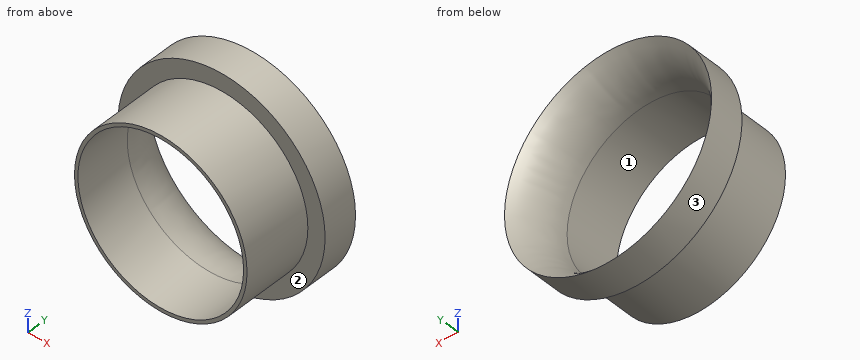
from build123d import *

# Parameters (mm, degrees)
F0_R     = 30
F1_DEPTH = 50
F2_R     = 30
F2_R_2   = 25
F3_DEPTH = 40
F4_R     = 24
F5_DEPTH = 60
F7_DEPTH = 20


# Not quite as in the source:
# - a fillet or chamfer that OpenCascade refuses, or shapes differently, is made with other operations: its cross-section is extruded or revolved along the edge and cut away or added


with BuildPart() as f1:
    # F0 (on Front) → F1 (new body)
    with BuildSketch(Plane.XZ):
        Circle(F0_R)
    extrude(amount=-F1_DEPTH)

    # F2 (on face) → F3 (cut)
    with BuildSketch(Plane.XZ):
        Circle(F2_R)
        Circle(F2_R_2, mode=Mode.SUBTRACT)
    extrude(amount=-F3_DEPTH, mode=Mode.SUBTRACT)

    # F4 (on face) → F5 (cut)
    with BuildSketch(Plane.XZ):
        Circle(F4_R)
    extrude(amount=-F5_DEPTH, mode=Mode.SUBTRACT)

    # F6: fillet of radius 18.8308657865 on 1 edges, made by hand

    # F6_s1 → F6_t2 (revolve, cut)
    with BuildSketch(Plane.XY):
        with BuildLine():
            ThreePointArc((30, 50), (25.5650351112, 43.7331811345), (24, 36.2170253777))
            Line((24, 36.2170253777), (23.6233826843, 36.2170253777))
            Line((23.6233826843, 36.2170253777), (23.6233826843, 50))
            Line((23.6233826843, 50), (24, 50.3766173157))
            ThreePointArc((24, 50.3766173157), (27, 50.3766173157), (29.7433826843, 50.2756594924))
            Line((29.7433826843, 50.2756594924), (30, 50))
        make_face()
    revolve(axis=Axis((0, 50, 0), (0, -1, 0)), mode=Mode.SUBTRACT)

    # F7 (cut): a face of the model
    f7_faces = [f1.faces().sort_by_distance(p)[0] for p in [
        (-24.2928932188, 0, 0),
    ]]
    extrude(f7_faces, amount=-F7_DEPTH, mode=Mode.SUBTRACT)


solid = f1.part
Geometry check sheet. Reference: the model listing, model coordinates, mm. Face numbers are marked on the shaded views. Round coordinates to 2 decimals unless told otherwise and drop trailing zeros. Loops run counter-clockwise (first coordinate to the right, second up) from the corner with the lowest first, then second, coordinate; pieces in that order, holes last.
Item 1: Cross-section at C-C on y = 34.25. Record the boundary of the cut face in (x, z).
Item 2: Cross-section at D-D on y = 38.25. Record the boundary of the cut face in (x, z).
Item 3: Mould release check, pull along Z, two halves, no side actions. Record for the marked faces 1, 2 and 3: pulls with the +Z half, pulls with the -Z half, needs draft (parallel to the pull), parting line crosses it, or undercut.
Item 4: Cross-section at A-A on z = 0. Record the boundary of the cut face in (x, y), then the cut area to 3 significant figures.
Item 5: Cross-section at B-B on x = 0. Record the boundary of the cut face in (y, z).
Item 6: Gauge pin test, flat ends, axial feed: pin 1 (6 mm diameter, centred on y = 42, z = -11.5, fed in from -X); pin 2 (2 mm diameter, centred on x = 4.5, y = 32.5, fed in from -Z); pin 3 (4 mm diameter, centred on x = -19.5, z = 9, fed in from -Y); pin 4 (5 mm diameter, centred on y = 46.5, z = 19, fed in from -X). Record the tip position at first contact, or that the pin passes through.
Item 7: Thickness scan on line 1 (Z direction, x = 0, y = 30.75); line 2 (Z direction, x = -12, y = 36.25); line 3 (X direction, y = 32.5, z = 15) (3 decimals). Record the ranges inside material, lowest first.
Answer sheet:
1. outline: circle Ø50 at (0, 0); hole circle Ø48 at (0, 0)
2. outline: circle Ø50 at (0, 0); hole circle Ø48.22 at (0, 0)
3. face 1: undercut
3. face 2: needs draft
3. face 3: parting line crosses it
4. outline: (-30, 40) - (-25, 40) - (-25, 20) - (-24, 20) - (-24, 36.22) arc R18.83 ccw to (-30, 50) - close; (24, 20) - (25, 20) - (25, 40) - (30, 40) - (30, 50) arc R18.83 ccw to (24, 36.22) - close
4. area: 109 mm2
5. outline: (20, -25) - (40, -25) - (40, -30) - (50, -30) arc R18.83 ccw to (36.22, -24) - (20, -24) - close; (20, 24) - (36.22, 24) arc R18.83 ccw to (50, 30) - (40, 30) - (40, 25) - (20, 25) - close
6. pin 1: stops at x = -28.77
6. pin 2: stops at z = -24.75
6. pin 3: passes through
6. pin 4: stops at x = -25.05
7. line 1: z = -25 to -24, 24 to 25
7. line 2: z = -21.93 to -20.78, 20.78 to 21.93
7. line 3: x = -20 to -18.735, 18.735 to 20
